Geometry check sheet. Reference: the model listing, model coordinates, mm. A direction names the side the tool comes from. Give positions to 0.01 mm unless a question says otherwise; leave off trailing zeros. Loops run counter-clockwise (first coordinate to the right, second up) from the corner with the lowest first, then second, coordinate; pieces in that order, holes last. Notation, with made-up numbers: (23.5, 36) -> (46.5, 36) arc R27 ccw to (46.5, 64) -> close; hole circle Ø1 at (26.25, 5). An arc over 180 degrees is marked (long way). One line per question, with ' | ' between items.
from build123d import *

# Parameters (mm, degrees)
F0_R     = 8
F0_R_2   = 3
F2_DEPTH = 2
F3_SIZE2 = 0.5
F3_SIZE  = 0.5
F1_W     = 0.8275934942
F1_H     = 12
F5_SIZE2 = 0.5
F5_SIZE  = 0.5


with BuildPart() as f2:
    # F0 (on Top) → F2 (new body)
    with BuildSketch(Plane.XY):
        Circle(F0_R)
        Circle(F0_R_2, mode=Mode.SUBTRACT)
    extrude(amount=F2_DEPTH)

    # F3
    f3_edges = [f2.edges().sort_by_distance(p)[0] for p in [
        (8, 0, 1),
        (-8, 0, 0),
        (-8, 0, 2),
    ]]
    chamfer(f3_edges, length=F3_SIZE, length2=F3_SIZE2)

    # F1 (on Front) → F4 (revolve)
    with BuildSketch(Plane.XZ):
        Polygon((-3, -18), (-3, 0), (-4.25, 0), (-4.25, -6), (-4.25, -18), align=None)
        with Locations((-4.6637967471, -12)):
            Rectangle(F1_W, F1_H)
    revolve(axis=Axis((0, 0, -9), (0, 0, -1)))

    # F5
    f5_edges = [f2.edges().sort_by_distance(p)[0] for p in [
        (5.077593, 0, -6),
        (5.077593, 0, -18),
    ]]
    chamfer(f5_edges, length=F5_SIZE, length2=F5_SIZE2)


solid = f2.part
Item 1: Sectioned sample at C-C (z = -3.5). Record the cut outline in (x, y), plus the area to 3 significant figures.
Result:
outline: circle Ø8.5 at (0, 0); hole circle Ø6 at (0, 0) | area: 28.5 mm2
Item 2: Scan lines: probe 1 along Y at (x, z) = (0, 0.9); probe 2 along Y at (x, z) = (0, -5.5); probe 3 along Z at (x, y) = (-4, 4.5). Record each from-to range of solid material in increasing order.
Result:
probe 1: -8 to -3, 3 to 8 | probe 2: -4.25 to -3, 3 to 4.25 | probe 3: 0 to 2
Item 3: Sectioned sample at A-A (y = 0). Record the cut outline in (x, z), plus the area to 3 significant figures.
Result:
outline: (-8, 0.5) -> (-7.5, 0) -> (-4.25, 0) -> (-4.25, -6) -> (-4.58, -6) -> (-5.08, -6.5) -> (-5.08, -17.5) -> (-4.58, -18) -> (-3, -18) -> (-3, 2) -> (-7.5, 2) -> (-8, 1.5) -> close; (3, -18) -> (4.58, -18) -> (5.08, -17.5) -> (5.08, -6.5) -> (4.58, -6) -> (4.25, -6) -> (4.25, 0) -> (7.5, 0) -> (8, 0.5) -> (8, 1.5) -> (7.5, 2) -> (3, 2) -> close | area: 83.9 mm2
Item 4: Release check for a two-part mould opening along Z. For faces 1 (the face through (-1, -3, -18)), 2 (the face through (4.03, -3.09, -11.92)), 3 (the face through (3.2, -3.2, 0)), 4 (the face through (3.2, 0.1, 2)) record: pulls with the +Z half, pulls with the -Z half, needs draft (parallel to the pull), parting line crosses it, or undercut.
Result:
face 1: pulls with the -Z half | face 2: needs draft | face 3: undercut | face 4: pulls with the +Z half
Item 5: Set-up check for faces 5 (the face through (-2.285, 3.584, -3.042)), 6 (the face through (-1.73, -7.81, 0.99)): record each of +Z, -Z, +X, -X, +Y, -Y from which the full face is reachable in a straight line by a thin tool's end or side.
Result:
face 5: none | face 6: +Z, -Z
Item 6: Depth check by flat-ended pin: pin 1 Ø8 at (x, y) = (0, 0) entering from +Z; pin 2 Ø8 at (x, z) = (-4.5, -7.5) entering from -Y; pin 3 Ø1.5 at (x, y) = (-0.5, -2) entering from +Z; pin 4 Ø1 at (y, z) = (4, -6) entering from +X. Enter the tip coordinate at first touch or a pass-through.
Result:
pin 1: z = 2 | pin 2: y = -5.05 | pin 3: through | pin 4: x = 3.33
